The listing builds one solid part. Answer for the finished solid, in the listing's coordinates (mm). Give positions to 0.01 mm unless a question says otherwise; leave off trailing zeros. Write each loop counter-clockwise with the first axis right and the second up, starting at its lowest first coordinate (ties: lowest second). Pieces come first, ordered by that corner, then holes. Notation, with made-up numbers: M 63,-33 L 96,-33 A18 ccw 96,-9 Z; hole C -10.75,-8 d5. An arc over 180 degrees is marked long. Answer as a JSON object with one key per item and string values.
```python
from build123d import *

# Parameters (mm, degrees)
F0_W     = 145.514168
F0_H     = 107.53687
F0_W_2   = 139.31417
F0_H_2   = 101.336874
F1_DEPTH = 11
F2_W     = 139.714174
F2_H     = 101.736876
F2_W_2   = 139.31417
F2_H_2   = 101.336874
F3_DEPTH = 10


with BuildPart() as f1:
    # F0 (on Top) → F1 (new body)
    with BuildSketch(Plane.XY):
        Rectangle(F0_W, F0_H)
        Rectangle(F0_W_2, F0_H_2, mode=Mode.SUBTRACT)
    extrude(amount=F1_DEPTH)

    # F2 (on Top) → F3 (cut)
    with BuildSketch(Plane.XY):
        Rectangle(F2_W, F2_H)
        Rectangle(F2_W_2, F2_H_2, mode=Mode.SUBTRACT)
    extrude(amount=F3_DEPTH, mode=Mode.SUBTRACT)


solid = f1.part
```
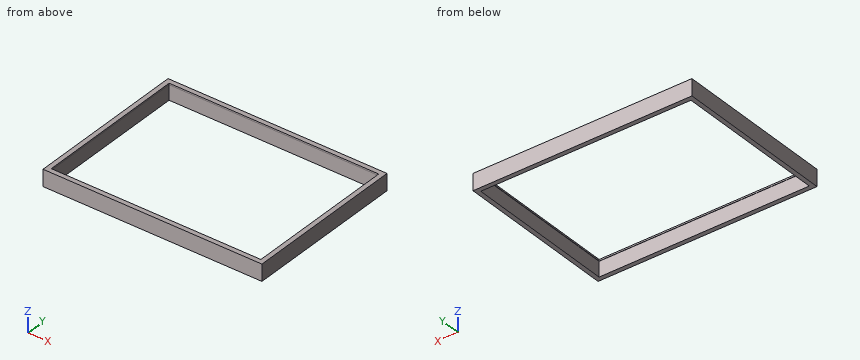
1. A cutting plane is placed at C-C, the plane z = 5. Give the vertices of the cut face in (x, y).
Verdict:
{"outline": "M -72.76,-53.77 L 72.76,-53.77 L 72.76,53.77 L -72.76,53.77 Z; hole M -69.86,-50.87 L 69.86,-50.87 L 69.86,50.87 L -69.86,50.87 Z"}
2. Consider line 1 along X through (y, z) = (-16.5, 4); line 2 along X through (y, z) = (46, 10.5); line 3 along Y through (x, z) = (-20.5, 8.5). Determine where each line is inside the solid, lowest interval first.
Verdict:
{"line 1": "x = -72.76 to -69.86, 69.86 to 72.76", "line 2": "x = -72.76 to -69.66, 69.66 to 72.76", "line 3": "y = -53.77 to -50.87, 50.87 to 53.77"}
3. A cutting plane is placed at A-A, the plane x = -34. Give the vertices of the cut face in (y, z).
Verdict:
{"outline": "M -53.77,0 L -50.87,0 L -50.87,10 L -50.67,10 L -50.67,11 L -53.77,11 Z; M 50.67,10 L 50.87,10 L 50.87,0 L 53.77,0 L 53.77,11 L 50.67,11 Z"}
4. A cutting plane is placed at B-B, the plane y = 47.5. Give the vertices of the cut face in (x, z).
Verdict:
{"outline": "M -72.76,0 L -69.86,0 L -69.86,10 L -69.66,10 L -69.66,11 L -72.76,11 Z; M 69.66,10 L 69.86,10 L 69.86,0 L 72.76,0 L 72.76,11 L 69.66,11 Z"}
